Here's how the part is built. I have some questions about the finished solid (model axes, mm). A direction names the side the tool comes from. Give positions to 0.01 mm unless a question says otherwise; leave off trailing zeros. Loops run counter-clockwise (first coordinate to the right, second up) from the corner with the lowest first, then second, coordinate; pieces in that order, holes last. Notation, with made-up numbers: (72.25, -38.75) -> (92.25, -38.75) arc R24 cw to (92.25, -22.75) -> close; hole circle Ø8 at (-29.75, 46). An arc over 180 degrees is marked (long way). Answer in a Markdown table with one row per item. Add a question column.
Item 1: We'd pull the mould along Y, two halves only. Please class faces 1 (the face through (4.12, 1.68, -1.67)), 2 (the face through (1.7, -3, 0)), 3 (the face through (4.14, 1.68, 1.65)), 4 (the face through (4.264, 6.77, 1.811)): released by +Y, released by -Y, zero draft, split by the parting line, or undercut.
Item 2: If we section it at C-C (y = 1.75): Write out the boundary of the cut face in (x, z) (3 decimals), then the cut area to 3 significant figures.
Item 3: Which directions (+Z, -Z, +X, -X, +Y, -Y) give clear straight access to the entire face, cutting with the end or side of a thin tool? Please do faces 5 (the face through (5.075, 7, 0)), 6 (the face through (-1, 2, 2.4)), 7 (the face through (4.264, 0.246, 1.811)), 8 (the face through (2.5, 1, 0)), 9 (the face through (-2.6, 7.1, 0.6)).
Item 4: If we section it at D-D (x = 4.25): Write out the boundary of the cut face in (y, z) (3 decimals).
Item 5: If I drill on line 1 (X direction, y = -0.4, z = 0) (3 decimals); line 2 (X direction, y = 0.25, z = 0) (3 decimals); line 3 (Z direction, x = 3, y = 4.75), over which ranges is the centre line in solid material (lowest first)?
Item 6: If we section it at A-A (y = -1.5): Write out the boundary of the cut face in (x, z) (3 decimals).
Item 7: If we section it at B-B (y = 8.25): Give the number of separate pieces and of enclosed holes in the cut face, then the cut area to 3 significant figures.
Item 8: For P1, Ø2.5, axis at x = 0, z = -0.5, coming from the -Y side; P2, Ø0.6, axis at x = -3.5, z = 0, coming from the -Y side; P3, Ø0.7, axis at x = -1, y = 2, coming from the +Z side, each with a flat end and sliding along its axis, tell me the tip position at first contact or that it passes through.
```python
from build123d import *

# Parameters (mm, degrees)
SHAPE_DEPTH         = 10.75
CUT_EXTRUDE1_DEPTH  = 6.75
CUT_EXTRUDE2_REACH  = 6
FILLET1_R           = 0.2
SKETCH4_R           = 1
BOSS_EXTRUDE2_DEPTH = 6.1
FILLET2_R           = 1
SKETCH5_W           = 0.2
SKETCH5_H           = 2
SKETCH5_W_2         = 2
SKETCH5_H_2         = 0.2
CUT_EXTRUDE3_DEPTH  = 6.75
CUT_EXTRUDE4_DEPTH  = 2.4
CUT_EXTRUDE5_DEPTH  = 1
SKETCH7_R           = 1.225
SKETCH7_R_2         = 0.625
BOSS_EXTRUDE3_DEPTH = 4
SKETCH9_W           = 1.225
SKETCH9_H           = 2.45
CUT_EXTRUDE6_DEPTH  = 2.3


with BuildPart() as part:
    # Sketch1 → Shape (new body)
    with BuildSketch(Plane(origin=(0, 0, 0), x_dir=(1, 0, 0), z_dir=(0, 1, 0))):
        Polygon((5.075, -1), (5.075, 1), (3.475, 2.6), (-5.075, 2.6), (-5.075, -2.6), (3.475, -2.6), align=None)
    extrude(amount=SHAPE_DEPTH)

    # Sketch2 → Cut-Extrude1 (cut)
    with BuildSketch(Plane(origin=(0, 10.75, 0), x_dir=(1, 0, 0), z_dir=(0, 1, 0))):
        Polygon((3.226471863, -2), (4.475, -0.751471863), (4.475, 0.751471863), (3.226471863, 2), (-4.475, 2), (-4.475, -2), align=None)
    extrude(amount=-CUT_EXTRUDE1_DEPTH, mode=Mode.SUBTRACT)

    # Sketch3 → Cut-Extrude2 (cut, up to next)
    with BuildSketch(Plane(origin=(0, 4, 0), x_dir=(1, 0, 0), z_dir=(0, 1, 0)), mode=Mode.PRIVATE) as cut_extrude2_sk1:
        with BuildLine():
            Line((-1.675378875, -1.6), (1.675378875, -1.6))
            ThreePointArc((1.675378875, -1.6), (0.7, 0), (1.675378875, 1.6))
            Line((1.675378875, 1.6), (-1.675378875, 1.6))
            ThreePointArc((-1.675378875, 1.6), (-0.963068312, 0.936931688), (-0.7, 0))
            ThreePointArc((-0.7, 0), (-0.963068312, -0.936931688), (-1.675378875, -1.6))
        make_face()
    cut_extrude2_tool1 = extrude(cut_extrude2_sk1.sketch, amount=-CUT_EXTRUDE2_REACH, mode=Mode.PRIVATE) & part.part
    add(cut_extrude2_tool1.solids().sort_by_distance((0, 4, 0))[0], mode=Mode.SUBTRACT)

    # Fillet1
    fillet1_edges = [part.edges().sort_by_distance(p)[0] for p in [
        (1.675378875, 2, 1.6),
        (-1.675378875, 2, 1.6),
        (-1.675378875, 2, -1.6),
        (1.675378875, 2, -1.6),
    ]]
    fillet(fillet1_edges, radius=FILLET1_R)

    # Sketch4 → Boss-Extrude2 (add)
    with BuildSketch(Plane(origin=(0, 4, 0), x_dir=(1, 0, 0), z_dir=(0, 1, 0))):
        with Locations((-2.5, 0)):
            Circle(SKETCH4_R)
        with Locations((2.5, 0)):
            Circle(SKETCH4_R)
    extrude(amount=BOSS_EXTRUDE2_DEPTH)

    # Fillet2
    fillet2_edges = [part.edges().sort_by_distance(p)[0] for p in [
        (-3.5, 10.1, 0),
        (1.5, 10.1, 0),
    ]]
    fillet(fillet2_edges, radius=FILLET2_R)

    # Sketch5 → Cut-Extrude3 (cut)
    with BuildSketch(Plane(origin=(0, 10.75, 0), x_dir=(1, 0, 0), z_dir=(0, 1, 0))):
        with Locations((-2.5, 0)):
            Rectangle(SKETCH5_W, SKETCH5_H)
        with Locations((-2.5, 0)):
            Rectangle(SKETCH5_W_2, SKETCH5_H_2)
        with Locations((2.5, 0)):
            Rectangle(SKETCH5_W_2, SKETCH5_H_2)
        with Locations((2.5, 0)):
            Rectangle(SKETCH5_W, SKETCH5_H)
    extrude(amount=-CUT_EXTRUDE3_DEPTH, mode=Mode.SUBTRACT)

    # Sketch6 → Cut-Extrude4 (cut)
    with BuildSketch(Plane(origin=(0, 0.5, 0), x_dir=(-1, 0, 0), z_dir=(0, -1, 0))):
        Polygon((-5.075, -1), (-3.475, -2.6), (5.075, -2.6), (5.075, 2.6), (-3.475, 2.6), (-5.075, 1), align=None)
        Polygon((-4.875, -0.917157288), (-3.392157288, -2.4), (4.875, -2.4), (4.875, 2.4), (-3.392157288, 2.4), (-4.875, 0.917157288), align=None, mode=Mode.SUBTRACT)
    extrude(amount=-CUT_EXTRUDE4_DEPTH, mode=Mode.SUBTRACT)

    # Sketch8 → Cut-Extrude5 (cut)
    with BuildSketch(Plane.XZ):
        Polygon((-4.475, -2), (-4.475, 2), (3.226471863, 2), (4.475, 0.751471863), (4.475, -0.751471863), (3.226471863, -2), align=None)
    extrude(amount=-CUT_EXTRUDE5_DEPTH, mode=Mode.SUBTRACT)

    # Sketch7 → Boss-Extrude3 (add)
    with BuildSketch(Plane.XZ.offset(-1)):
        with Locations((-2.5, 0)):
            Circle(SKETCH7_R)
        with Locations((-2.5, 0)):
            Circle(SKETCH7_R_2, mode=Mode.SUBTRACT)
        with Locations((2.5, 0)):
            Circle(SKETCH7_R)
        with Locations((2.5, 0)):
            Circle(SKETCH7_R_2, mode=Mode.SUBTRACT)
    extrude(amount=BOSS_EXTRUDE3_DEPTH)

    # Sketch9 → Cut-Extrude6 (cut)
    with BuildSketch(Plane.XZ.offset(3)):
        with Locations((-3.1125, 0)):
            Rectangle(SKETCH9_W, SKETCH9_H)
        with Locations((3.1125, 0)):
            Rectangle(SKETCH9_W, SKETCH9_H)
    extrude(amount=-CUT_EXTRUDE6_DEPTH, mode=Mode.SUBTRACT)


solid = part.part
```
Recorded:
| question | item | result |
|---|---|---|
| 1 | face 1 | undercut |
| 1 | face 2 | released by -Y |
| 1 | face 3 | undercut |
| 1 | face 4 | zero draft |
| 2 | outline | (-4.875, -2.4) -> (3.392, -2.4) -> (4.875, -0.917) -> (4.875, 0.917) -> (3.392, 2.4) -> (-4.875, 2.4) -> close; hole (-1.215, -1.26) arc R0.2 ccw to (-1.072, -1.6) -> (1.072, -1.6) arc R0.2 ccw to (1.215, -1.26) arc R1.8 cw to (1.215, 1.26) arc R0.2 ccw to (1.072, 1.6) -> (-1.072, 1.6) arc R0.2 ccw to (-1.215, 1.26) arc R1.8 cw to start |
| 2 | area | 38.6 mm^2 |
| 3 | face 5 | +Z, -Z, +X, +Y, -Y |
| 3 | face 6 | +Z, +X, -X |
| 3 | face 7 | +Z, +X, +Y, -Y |
| 3 | face 8 | -Y |
| 3 | face 9 | +Y |
| 4 | outline | (0, -1.825) -> (0.5, -1.825) -> (0.5, -1.542) -> (2.9, -1.542) -> (2.9, -1.825) -> (10.75, -1.825) -> (10.75, -0.976) -> (4, -0.976) -> (4, 0.976) -> (10.75, 0.976) -> (10.75, 1.825) -> (2.9, 1.825) -> (2.9, 1.542) -> (0.5, 1.542) -> (0.5, 1.825) -> (0, 1.825) -> (0, 0.976) -> (1, 0.976) -> (1, -0.976) -> (0, -0.976) -> close |
| 5 | line 1 | x = -3.725 to -3.125, -1.875 to -1.275, 1.275 to 1.875, 3.125 to 3.725 |
| 5 | line 2 | x = -5.075 to -4.475, -3.725 to -3.125, -1.875 to -1.275, 1.275 to 1.875, 3.125 to 3.725, 4.475 to 5.075 |
| 5 | line 3 | z = -2.6 to -2, -0.87 to -0.1, 0.1 to 0.87, 2 to 2.6 |
| 6 | outline | (-2.5, -1.225) arc R1.225 ccw to (-2.5, 1.225) -> (-2.5, 0.625) arc R0.625 cw to (-2.5, -0.625) -> close; (2.5, -1.225) -> (2.5, -0.625) arc R0.625 cw to (2.5, 0.625) -> (2.5, 1.225) arc R1.225 ccw to start |
| 7 | separate pieces | 9 |
| 7 | enclosed holes | 1 |
| 7 | area | 20.7 mm^2 |
| 8 | P1 | stops at y = 1 |
| 8 | P2 | stops at y = -0.7 |
| 8 | P3 | stops at z = 2.4 |
